Source: CAD feature listing. Evaluate the final solid. Frame: model axes, mm. A direction names the side the tool comes from. Round coordinates to 2 decimals unless told otherwise and drop trailing zeros. Loops run counter-clockwise (first coordinate to the right, second up) from the corner with the lowest first, then second, coordinate; pieces in that order, holes last.
(1) Material intervals for probe 1 along Y at (x, z) = (25, 2.3); probe 2 along X at (y, z) = (3.5, 2.7); probe 3 along Z at (x, y) = (25.5, 2), sorted ascending.
(2) Set-up query: faces 1 (the cylindrical face through (18.147, 6.304, 0.401)), 2 (the cylindrical face through (19.34, 1.442, 2.01)). Return all of +Z, -Z, +X, -X, +Y, -Y with unobstructed straight access to the full face (end or side cutting, diameter ignored); none if empty.
(3) Section B-B, the plane x = 25. Return the cut outline in (y, z) (3 decimals).
(4) Section A-A, the plane y = 1.25. Return the cut outline in (x, z) (3 decimals).
(5) Section D-D, the plane x = 17. Return the cut outline in (y, z) (3 decimals).
(6) First-contact query: pin 1 Ø1.9 at (y, z) = (5.5, 2) entering from +X; pin 2 Ø5 at (x, y) = (9.5, 3) entering from -Z; pin 3 Ø1.5 at (x, z) = (25.5, 1) entering from -Y; pin 4 Ø1.5 at (x, y) = (14.92, 0.53) entering from -Z. Flat tips, straight axial feed; report the tip coordinate or a pass-through.
(7) Section C-C, the plane z = 1.7. Count the separate pieces of the cut face and the enclosed holes in it, plus the area to 3 significant figures.
(8) Mould query, pull axis Z, two halves, no side actions, for faces 3 (the flat face through (15, 3, 0)), 4 (the flat face through (19, 3, 0.813)), 5 (the cylindrical face through (30.201, 2.333, 0.412)), 6 (the cylindrical face through (4.01, 3.49, 2.37)). Classes: pulls with the +Z half, pulls with the -Z half, needs draft (parallel to the pull), parting line crosses it, or undercut.
Autodesk Inventor part; units mm, degrees
ref_plane "YZ Plane" through (0, 0, 0) normal (1, 0, 0) x (0, 1, 0)
ref_plane "XZ Plane" through (0, 0, 0) normal (0, 1, 0) x (-1, 0, 0)
ref_plane "XY Plane" through (0, 0, 0) normal (0, 0, 1) x (1, 0, 0)
sketch "Sketch1" plane through (0, 0, 0) normal (0, 0, 1) x (1, 0, 0)
  line L0 (0, 0) -> (0, -93.6625)
  line L1 (0, 0) -> (0, 7.9375)
  arc A0 (31.3961, 2.9648) -> (0, 7.9375) centre (0, -93.6625) ccw
  arc A1 (28.9433, -4.5842) -> (0, 0) centre (0, -93.6625) ccw
  line L2 (0, -93.6625) -> (35.0444, 14.1931)
  line L3 (14.9183, 0.5277) -> (0, -93.6625)
  line L4 (14.9183, 0.5277) -> (26.5201, -1.3098)
  circle A2 centre (14.9183, 0.5277) radius 1.27
  line L5 (0, -93.6625) -> (24.6821, -1.5477)
  line L6 (24.6821, -1.5477) -> (28.1101, -2.4662)
  circle A3 centre (24.6821, -1.5477) radius 1.27
  dimension "d0" = 93.6625
  dimension "d1" = 7.9375
  dimension "d2" = 18
  dimension "d5" = 9
  dimension "d28" = 95.3643
  dimension "d29" = 2.54
  dimension "d32" = 6
  dimension "d33" = 95.3643
  dimension "d34" = 2.54
extrude "Extrusion2" add sketch "Sketch1" along normal blind 3.175 contours L1 A0 L2 A1 L5 A3 L4 A2 L3 | L3 A2 L4 A3 L5 A1 | A2 L4 L3 | L3 L4 A2 | A3 L4 L6 L5 | L5 L6 A3 | A3 L4
sketch "Sketch3" plane through (0, 0, 0) normal (-1, 0, 0) x (0, 0, 1)
  line L0 (3.175, 0) -> (3.175, 7.9375)
  line L1 (0, 0) -> (3.175, 0)
  line L2 (0, 7.9375) -> (3.175, 7.9375)
  line L3 (3.175, 7.9375) -> (3.175, 3.048)
  line L4 (3.175, 3.048) -> (0, 3.048)
  line L5 (0, 3.048) -> (0, 7.9375)
  dimension "d13" = 3.048
extrude "Extrusion3" cut sketch "Sketch3" against normal blind 8.128
sketch "Sketch4" plane through (8.128, 0, 0) normal (-1, 0, 0) x (0, 0, 1)
  line L0 (0, 3.048) -> (0, 7.6119)
  line L1 (0, 3.048) -> (3.175, 3.048)
  line L2 (3.175, 7.6119) -> (3.175, 3.048)
  line L3 (3.175, 7.6119) -> (0.8128, 7.6119)
  line L4 (0.8128, 7.6119) -> (0.8128, 3.048)
  line L5 (0.8128, 3.048) -> (3.175, 3.048)
  line L6 (3.175, 3.048) -> (3.175, 7.6119)
  point P0 (0, 0)
  dimension "d16" = 0.8128
sketch3d "3D Sketch1"
  arc A0 (8.128, 7.6119, 0) -> (31.3961, 2.9648, 0) centre (0, -93.6625, 0) ccw
sweep "Sweep1" cut profiles "Sketch4" path "3D Sketch1"
sketch "Sketch5" plane through (0, 3.048, 3.175) normal (0, 1, 0) x (1, 0, 0)
  line L0 (0, 3.175) -> (8.128, 3.175)
  line L1 (8.128, 3.175) -> (8.128, 0)
  line L2 (8.128, 0) -> (0, 0)
  line L3 (0, 0) -> (0, 3.175)
extrude "Extrusion4" add sketch "Sketch5" along normal blind 4.8895
sketch "Sketch6" plane through (0, 0, 0) normal (-1, 0, 0) x (0, 0, 1)
  line L0 (0, 7.9375) -> (3.175, 7.9375)
  line L1 (3.175, 7.9375) -> (3.175, 8.7188)
  line L2 (3.175, 8.7188) -> (0, 8.7188)
  line L3 (0, 8.7188) -> (0, 7.9375)
sweep "Sweep2" cut profiles "Sketch6" path "Sketch1" path curves L1 A0
sketch "Sketch7" plane through (0, 0, 0) normal (-1, 0, 0) x (0, 0, 1)
  line L0 (0, 0) -> (3.175, 0)
  circle A0 centre (1.905, 4.3942) radius 1.016
  line L1 (3.175, 0) -> (3.175, 7.9375)
  dimension "d21" = 2.032
  dimension "d22" = 4.3942
  dimension "d25" = 1.27
extrude "Extrusion5" cut sketch "Sketch7" against normal blind 50.8
sketch "Sketch8" plane through (8.128, 3.048, 3.175) normal (1, 0, 0) x (0, 0, -1)
  circle A0 centre (1.27, 1.3462) radius 1.016
  line L0 (2.3622, 4.5639) -> (0, 4.5639)
  line L1 (0, 0) -> (0, 4.5639)
  line L2 (2.3622, 0) -> (0, 0)
  line L3 (2.3622, 0) -> (2.3622, 4.5639)
  point P0 (3.175, -3.048)
  dimension "d26" = 1.3462
fillet "Fillet1" radius 3.175 1 edges at (31.3961, 2.9648, 0.4064)
extrude "Extrusion9" cut sketch "Sketch1" along normal blind 12.7 contours A2 L4 L3 | L3 L4 A2 | A3 L4 L6 L5 | L5 L6 A3 | A3 L4
sketch "Sketch10" plane through (0, 0, 3.175) normal (0, 0, 1) x (1, 0, 0)
  circle A0 centre (24.6821, -1.5477) radius 1.27
  circle A1 centre (14.9183, 0.5277) radius 1.27
  arc A2 (8.128, 7.6119) -> (0, 7.9375) centre (0, -93.6625) ccw
  line L0 (0, 0) -> (0, 7.9375)
  arc A3 (28.9433, -4.5842) -> (0, 0) centre (0, -93.6625) ccw
  line L1 (29.9905, -1.3611) -> (28.9433, -4.5842)
  arc A4 (29.9905, -1.3611) -> (8.128, 3.048) centre (0, -93.6625) ccw
  line L2 (8.128, 3.048) -> (8.128, 7.6119)
  dimension "d45" = 14.9183
  dimension "d46" = 24.6821
  dimension "d47" = 0.5277
  dimension "d48" = 1.5477
equation "\"d33\" = d28"
properties part number "FiberClamper_v2"
Output values:
1. probe 1: y = -3.4 to -2.78, -0.32 to 0.11
1. probe 2: x = 0 to 8.13
1. probe 3: z = 0 to 0.81
2. face 1: +Z, -Z, +X, +Y
2. face 2: +Z, +X, +Y
3. outline: (-3.398, 0) - (-2.777, 0) - (-2.777, 3.175) - (-3.398, 3.175) - close; (-0.318, 0) - (4.814, 0) - (4.814, 0.813) - (0.114, 0.813) - (0.114, 3.175) - (-0.318, 3.175) - close
4. outline: (0, 0) - (13.874, 0) - (13.874, 3.175) - (0, 3.175) - close; (15.963, 0) - (30.533, 0) - (30.533, 0.813) - (20.263, 0.813) - (20.263, 3.175) - (15.963, 3.175) - close
5. outline: (-1.556, 0) - (6.505, 0) - (6.505, 0.813) - (1.888, 0.813) - (1.888, 3.175) - (-1.556, 3.175) - close
6. pin 1: stops at x = 8.13
6. pin 2: stops at z = 0
6. pin 3: stops at y = -3.75
6. pin 4: passes through
7. separate pieces: 2
7. enclosed holes: 2
7. area: 112 mm2
8. face 3: pulls with the -Z half
8. face 4: pulls with the +Z half
8. face 5: needs draft
8. face 6: undercut
